from build123d import *

# Parameters (mm, degrees)
BOSS_EXTRUDE1_DEPTH = 7
BOSS_EXTRUDE2_DEPTH = 1
SKETCH3_W           = 10.974831657
SKETCH3_H           = 5.618667726
CUT_EXTRUDE1_DEPTH  = 4
CUT_EXTRUDE2_DEPTH  = 3
CUT_EXTRUDE3_DEPTH  = 1


with BuildPart() as part:
    # Sketch1 → Boss-Extrude1 (new body)
    with BuildSketch(Plane.XY):
        with BuildLine():
            Line((-7, -2), (-7, -5))
            Line((-7, -5), (7, -5))
            Line((7, -5), (7, -2))
            ThreePointArc((7, -2), (6.414213562, -0.585786438), (5, 0))
            ThreePointArc((5, 0), (3.585786438, 0.585786438), (3, 2))
            ThreePointArc((3, 2), (0, 5), (-3, 2))
            ThreePointArc((-3, 2), (-3.585786438, 0.585786438), (-5, 0))
            ThreePointArc((-5, 0), (-6.414213562, -0.585786438), (-7, -2))
        make_face()
        with BuildLine():
            Line((-2, 0), (-2, 2))
            ThreePointArc((-2, 2), (0, 4), (2, 2))
            Line((2, 2), (2, 0))
            ThreePointArc((2, 0), (0, -2), (-2, 0))
        make_face(mode=Mode.SUBTRACT)
    extrude(amount=BOSS_EXTRUDE1_DEPTH)

    # Sketch2 → Boss-Extrude2 (add)
    with BuildSketch(Plane(origin=(0, 0, 0), x_dir=(-1, 0, 0), z_dir=(0, 0, -1))):
        with BuildLine():
            ThreePointArc((7, -2), (6.880189856, -1.318174432), (6.535113895, -0.718038484))
            Line((6.535113895, -0.718038484), (6.410807281, -0.582388341))
            ThreePointArc((6.410807281, -0.582388341), (5.763143722, -0.151321645), (5, 0))
            ThreePointArc((5, 0), (3.585786438, 0.585786438), (3, 2))
            ThreePointArc((3, 2), (2.851719503, 2.931501945), (2.421536084, 3.77092151))
            ThreePointArc((2.421536084, 3.77092151), (0, 5), (-2.421536084, 3.77092151))
            ThreePointArc((-2.421536084, 3.77092151), (-2.851719503, 2.931501945), (-3, 2))
            ThreePointArc((-3, 2), (-3.585786438, 0.585786438), (-5, 0))
            ThreePointArc((-5, 0), (-5.763143722, -0.151321645), (-6.410807281, -0.582388341))
            Line((-6.410807281, -0.582388341), (-6.535113895, -0.718038484))
            ThreePointArc((-6.535113895, -0.718038484), (-6.880189856, -1.318174432), (-7, -2))
            Line((-7, -2), (-7, -5))
            Line((-7, -5), (7, -5))
            Line((7, -5), (7, -2))
        make_face()
        with BuildLine():
            ThreePointArc((2, 0), (0, -2), (-2, 0))
            Line((-2, 0), (-2, 2))
            ThreePointArc((-2, 2), (0, 4), (2, 2))
            Line((2, 2), (2, 0))
        make_face(mode=Mode.SUBTRACT)
        with BuildLine():
            ThreePointArc((5, 0), (5.763143722, -0.151321645), (6.410807281, -0.582388341))
            Line((6.410807281, -0.582388341), (2.421536084, 3.77092151))
            ThreePointArc((2.421536084, 3.77092151), (2.851719503, 2.931501945), (3, 2))
            ThreePointArc((3, 2), (3.585786438, 0.585786438), (5, 0))
        make_face()
        with BuildLine():
            ThreePointArc((-3, 2), (-2.851719503, 2.931501945), (-2.421536084, 3.77092151))
            Line((-2.421536084, 3.77092151), (-6.410807281, -0.582388341))
            ThreePointArc((-6.410807281, -0.582388341), (-5.763143722, -0.151321645), (-5, 0))
            ThreePointArc((-5, 0), (-3.585786438, 0.585786438), (-3, 2))
        make_face()
    extrude(amount=-BOSS_EXTRUDE2_DEPTH)

    # Sketch3 → Cut-Extrude1 (cut)
    with BuildSketch(Plane.XY.offset(7)):
        with Locations((0.487415829, 2.809333863)):
            Rectangle(SKETCH3_W, SKETCH3_H)
    extrude(amount=-CUT_EXTRUDE1_DEPTH, mode=Mode.SUBTRACT)

    # Sketch4 → Cut-Extrude2 (cut)
    with BuildSketch(Plane.XY.offset(7)):
        with BuildLine():
            Line((3, 2), (3, 0))
            ThreePointArc((3, 0), (0, -3), (-3, 0))
            Line((-3, 0), (-3, 2))
            ThreePointArc((-3, 2), (0, 5), (3, 2))
        make_face()
    extrude(amount=-CUT_EXTRUDE2_DEPTH, mode=Mode.SUBTRACT)

    # Sketch5 → Cut-Extrude3 (cut)
    with BuildSketch(Plane.XY.offset(7)):
        Polygon((0, -3), (-4, -3), (-5, -4), (-5, -5), (-7, -5), (-7, 0), (0, 0), align=None)
    extrude(amount=-CUT_EXTRUDE3_DEPTH, mode=Mode.SUBTRACT)


solid = part.part
The model under review builds one solid part; all positions refer to its coordinate system, in mm. A direction names the side the tool comes from. Coordinates: 2 decimals unless noted, no trailing zeros. Loops run counter-clockwise (first coordinate to the right, second up) from the corner with the lowest first, then second, coordinate; pieces in that order, holes last.
(1) Consider section B-B, the plane y = -0.25. Give the boundary of the cut face in (x, z).
Determined:
outline: (-6.11, 0) - (-1.98, 0) - (-1.98, 4) - (-2.99, 4) - (-2.99, 6) - (-5.97, 6) - (-5.97, 1) - (-6.11, 1) - close; (1.98, 0) - (6.11, 0) - (6.11, 1) - (5.97, 1) - (5.97, 7) - (2.99, 7) - (2.99, 4) - (1.98, 4) - close
(2) Consider section C-C, the plane y = -2.5. Give the boundary of the cut face in (x, z).
Determined:
outline: (-7, 0) - (7, 0) - (7, 7) - (1.66, 7) - (1.66, 4) - (-1.66, 4) - (-1.66, 6) - (-7, 6) - close
(3) Consider section A-A, the plane z = 5.25. Give the boundary of the cut face in (x, y).
Determined:
outline: (-7, -5) - (7, -5) - (7, -2) arc R2 ccw to (5, 0) - (3, 0) arc R3 cw to (-3, 0) - (-5, 0) arc R2 ccw to (-7, -2) - close
(4) Consider section D-D, the plane y = 1. Give the boundary of the cut face in (x, z), plus the area to 3 significant figures.
Determined:
outline: (-4.96, 0) - (-2, 0) - (-2, 3) - (-3.27, 3) - (-3.27, 1) - (-4.96, 1) - close; (2, 0) - (4.96, 0) - (4.96, 1) - (3.27, 1) - (3.27, 3) - (2, 3) - close
area: 11.0 mm2
(5) Draft analysis for pull direction X (two halves, no side actions). For faces 1 (the flat face through (-4.444, 1.564, 0.493)), 2 (the flat face through (1, 4, 3)), 3 (the flat face through (2, 1, 1)), state which applies: +X half, -X half, draft (parallel to the pull), parting line (faces both ways), or undercut.
Determined:
face 1: -X half
face 2: draft
face 3: undercut
(6) Insertion check: P1, Ø1.5, axis at x = -3, z = 4, coming from the +Y side; P2, Ø5.5, axis at x = -0.5, y = 1.5, coming from the +Z side; P3, Ø0.5, axis at y = -4.5, z = 6.5, coming from the -X side; P4, Ø2, axis at x = -5, y = 2.5, coming from the +Z side. Each pin has a flat end and moves straight along its axis. Give the tip position at first contact, or say it passes through.
Determined:
P1: stops at y = 0
P2: stops at z = 4
P3: stops at x = -5
P4: passes through
(7) Tool access review of faces 4 (the cylindrical face through (1.088, -2.796, 5.188)), 5 (the flat face through (-4, 0, 5)), 6 (the flat face through (-5, -2, 6)), 7 (the flat face through (-5, -4.5, 6.5)): name each direction out of +Z, -Z, +X, -X, +Y, -Y from which nothing blocks a thin tool from reaching the whole face with its end or side.
Determined:
face 4: +Z, +Y
face 5: +Z, +X, -X, +Y
face 6: +Z, -X, +Y
face 7: +Z, -X, +Y, -Y
(8) Wall thickness on L1, parallel to Y at x = -2.25, z = 3.5; L2, parallel to X at y = -0.5, z = 2.25; L3, parallel to Z at x = -2.5, y = 1.25: over which ranges is each line inside the solid? List them lowest first.
Determined:
L1: y = -5 to 0
L2: x = -6.32 to -1.94, 1.94 to 6.32
L3: z = 0 to 3
